Answer from the drawing. Dimensions are ordinates in mm from the lowest x, y and z of the part. Coordinates: 2 decimals unless noted, no trailing zeros. Write each loop counter-clockwise with the first axis right and the second up, starting at its lowest first coordinate (ties: lowest second). Pieces come first, ordered by that corner, then holes. Notation, with made-up numbers: (-38, 56.5) -> (-5, 56.5) arc R5 ccw to (-5, 63.5) -> close; hole circle Ø3 at (56.25, -6.5). An arc over 180 degrees is marked (long way). One line per item, written item: value. Start each with the question number.
1. Find section C-C, the plane x = 131.5. Write down the section's boundary in (y, z).
2. Consider line 1 along X through (y, z) = (110, 1.7); line 2 along Y through (x, z) = (109, 2.05); line 3 along Y through (x, z) = (107.5, 0.25). Determine where each line is inside the solid, lowest interval first.
3. Find section A-A, the plane y = 170. Write down the section's boundary in (x, z).
4. Find section D-D, the plane x = 109. Write down the section's boundary in (y, z), and give its area (3 significant figures).
5. Find section B-B, the plane z = 3.95. Write down the section's boundary in (x, y).
6. Given P1, Ø3, axis at y = 225.5, z = 2.5, coming from the +X side; P2, Ø2, axis at x = 69.5, z = 2, coming from the -Y side; P3, Ø3, axis at x = 85, z = 0.5, coming from the +Y side, each flat-ended and moving along its own axis, determine where each tip first touches the part or whether it passes through.
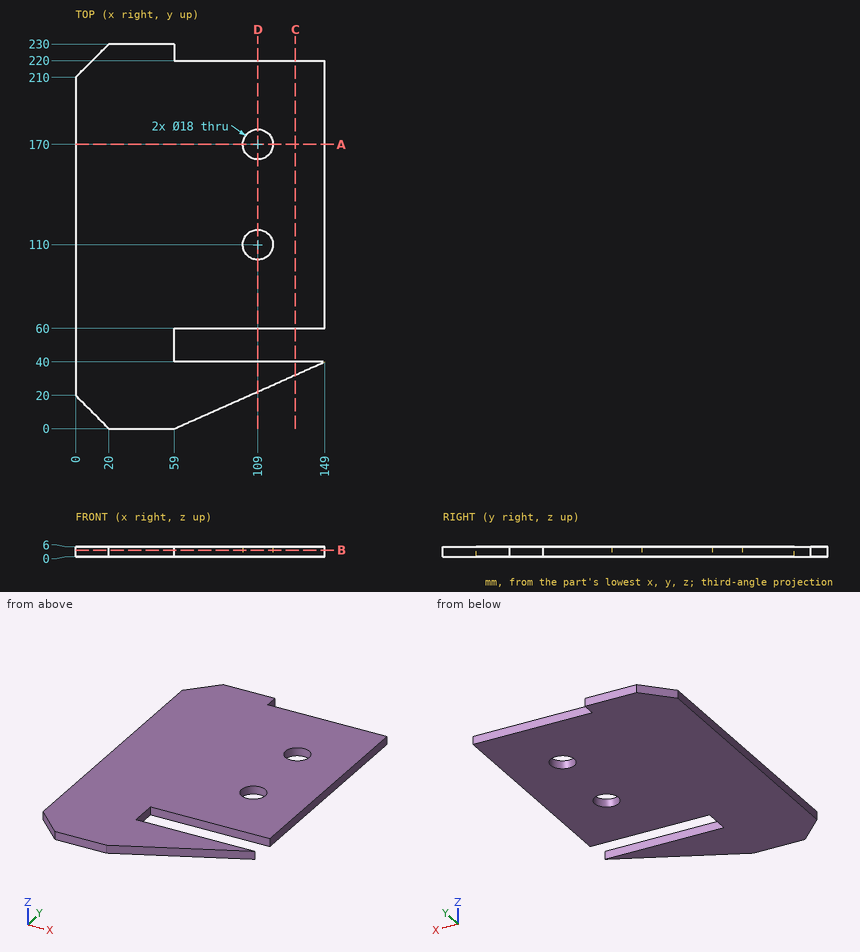
Answer block:
1. outline: (32.22, 0) -> (40, 0) -> (40, 6) -> (32.22, 6) -> close; (60, 0) -> (220, 0) -> (220, 6) -> (60, 6) -> close
2. line 1: x = 0 to 100, 118 to 149
2. line 2: y = 22.22 to 40, 60 to 101, 119 to 161, 179 to 220
2. line 3: y = 21.56 to 40, 60 to 101.13, 118.87 to 161.13, 178.87 to 220
3. outline: (0, 0) -> (100, 0) -> (100, 6) -> (0, 6) -> close; (118, 0) -> (149, 0) -> (149, 6) -> (118, 6) -> close
4. outline: (22.22, 0) -> (40, 0) -> (40, 6) -> (22.22, 6) -> close; (60, 0) -> (101, 0) -> (101, 6) -> (60, 6) -> close; (119, 0) -> (161, 0) -> (161, 6) -> (119, 6) -> close; (179, 0) -> (220, 0) -> (220, 6) -> (179, 6) -> close
4. area: 851 mm2
5. outline: (0, 20) -> (20, 0) -> (59, 0) -> (149, 40) -> (59, 40) -> (59, 60) -> (149, 60) -> (149, 220) -> (59, 220) -> (59, 230) -> (20, 230) -> (0, 210) -> close; hole circle Ø18 at (109, 110); hole circle Ø18 at (109, 170)
6. P1: stops at x = 59
6. P2: stops at y = 4.22
6. P3: stops at y = 220
